```python
from build123d import *

# Parameters (mm, degrees)
SKETCH1_R           = 25
SKETCH1_R_2         = 4.1
BOSS_EXTRUDE1_DEPTH = 12
SKETCH2_R           = 11
CUT_EXTRUDE1_DEPTH  = 5
SKETCH3_R           = 11.05
CUT_EXTRUDE2_DEPTH  = 5


with BuildPart() as part:
    # Sketch1 → Boss-Extrude1 (new body)
    with BuildSketch(Plane(origin=(0, 0, 0), x_dir=(1, 0, 0), z_dir=(0, 1, 0))):
        with Locations(Location((0, 0, 0), (0, 0, 270))):
            Circle(SKETCH1_R)
        with Locations(Location((0, 0, 0), (0, 0, 270))):
            Circle(SKETCH1_R_2, mode=Mode.SUBTRACT)
    extrude(amount=BOSS_EXTRUDE1_DEPTH)

    # Sketch2 → Cut-Extrude1 (cut)
    with BuildSketch(Plane(origin=(0, 12, 0), x_dir=(1, 0, 0), z_dir=(0, 1, 0))):
        with Locations(Location((0, 0, 0), (0, 0, 270))):
            Circle(SKETCH2_R)
    extrude(amount=-CUT_EXTRUDE1_DEPTH, mode=Mode.SUBTRACT)

    # Sketch3 → Cut-Extrude2 (cut)
    with BuildSketch(Plane.XZ):
        with Locations(Location((0, 0, 0), (0, 0, 270))):
            Circle(SKETCH3_R)
    extrude(amount=-CUT_EXTRUDE2_DEPTH, mode=Mode.SUBTRACT)


solid = part.part
```
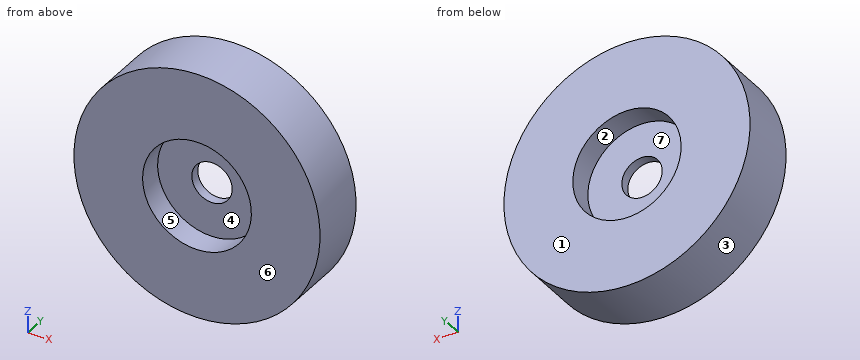
Work out the finished part from the listing and answer in its coordinate system (mm). Face numbers are marked on the shaded views. A direction names the side the tool comes from. Round coordinates to 2 decimals unless told otherwise and drop trailing zeros. Write each loop counter-clockwise with the first axis right and the second up, starting at its lowest first coordinate (ties: lowest second). Pieces come first, ordered by that corner, then holes.
1) A cutting plane is placed at C-C on y = 2.75. Determine the outline of the cut face in (x, z).
2) A cutting plane is placed at B-B on z = 0. Determine the outline of the cut face in (x, y), and give its area (3 significant figures).
3) Determine the mould class of the marked faces 1, 2, 3 and 4 for opening direction X: pulls with the +X half, pulls with the -X half, needs draft (parallel to the pull), parting line crosses it, or undercut.
4) Flat-ended cylindrical pins translate along their axes: P1, Ø11, axis at x = -1.5, z = -5, coming from the +Y side; P2, Ø3, axis at y = 1, z = -17, coming from the -X side; P3, Ø4, axis at x = -15, y = 5, coming from the -Z side; P4, Ø10, axis at x = -11.5, z = -11.5, coming from the -Y side. Find the tip coordinate at first contact, or state that the pin passes through.
5) Which of the six approach directions +Z, -Z, +X, -X, +Y, -Y give full straight-line access (tool end or side, diameter ignored) to the marked faces 5, 6 and 7?
6) A cutting plane is placed at A-A on x = 0. Determine the outline of the cut face in (y, z).
7) Consider probe 1 along X at (y, z) = (7.75, 0.5) (3 decimals); probe 2 along X at (y, z) = (6.2, 0); probe 3 along Z at (x, y) = (5, 1.5). Determine where each line is inside the solid, lowest interval first.
8) A cutting plane is placed at D-D on z = -5.5. Determine the outline of the cut face in (x, y).
Entries:
1. outline: circle Ø50 at (0, 0); hole circle Ø22.1 at (0, 0)
2. outline: (-25, 0) - (-11.05, 0) - (-11.05, 5) - (-4.1, 5) - (-4.1, 7) - (-11, 7) - (-11, 12) - (-25, 12) - close; (4.1, 5) - (11.05, 5) - (11.05, 0) - (25, 0) - (25, 12) - (11, 12) - (11, 7) - (4.1, 7) - close
2. area: 363 mm2
3. face 1: needs draft
3. face 2: undercut
3. face 3: parting line crosses it
3. face 4: undercut
4. P1: stops at y = 7
4. P2: stops at x = -19.62
4. P3: stops at z = -21.35
4. P4: stops at y = 0
5. face 5: -Y
5. face 6: +Z, -Z, +X, -X, -Y
5. face 7: +Y
6. outline: (0, -25) - (12, -25) - (12, -11) - (7, -11) - (7, -4.1) - (5, -4.1) - (5, -11.05) - (0, -11.05) - close; (0, 11.05) - (5, 11.05) - (5, 4.1) - (7, 4.1) - (7, 11) - (12, 11) - (12, 25) - (0, 25) - close
7. probe 1: x = -24.995 to -10.989, 10.989 to 24.995
7. probe 2: x = -25 to -4.1, 4.1 to 25
7. probe 3: z = -24.49 to -9.85, 9.85 to 24.49
8. outline: (-24.39, 0) - (-9.58, 0) - (-9.58, 5) - (9.58, 5) - (9.58, 0) - (24.39, 0) - (24.39, 12) - (9.53, 12) - (9.53, 7) - (-9.53, 7) - (-9.53, 12) - (-24.39, 12) - close
